Input: dimensioned drawing with shaded views. Units: mm. Origin: part minimum x, y, z. A direction names the side the tool comes from. Give positions to 0.01 mm unless a question says otherwise; leave off trailing zeros. Order: outer loops, then holes, each group sorted by start corner. A loop starts at its lowest first (then second) coordinate and runs counter-clockwise, first axis right, second up. Notation, with made-up numbers: M 7.5,-12 L 13.5,-12 A17 cw 13.5,13 Z; hole C 22,67.5 d4. An arc over 180 degrees is marked long. Answer in a Markdown table with one row per item. Add a question column.
(1) Section query D-D, the plane z = 6. Return loops of the section in (x, y), plus the area to 3 significant figures.
(2) Pin query (flat end, axial travel): P1, Ø15, axis at y = 26, z = 33.5, coming from the +X side; P2, Ø2, axis at y = 29.5, z = 10, coming from the +X side; P3, Ø1, axis at x = 41.5, y = 20.5, coming from the +Z side; P4, Ø6, axis at x = 41, z = 25, coming from the -Y side. Return the tip coordinate at first contact, or that it passes through.
(3) Section query C-C, the plane y = 17.34. Return loops of the section in (x, z), plus the area to 3 significant figures.
(4) Section query A-A, the plane z = 42. Return loops of the section in (x, y).
(5) Section query B-B, the plane x = 30.5. Return loops of the section in (y, z), plus the area to 3 significant figures.
(6) Set-up query: the marked faces 1 and 2. Return all of +Z, -Z, +X, -X, +Y, -Y with unobstructed straight access to the full face (end or side cutting, diameter ignored); none if empty.
(7) Mould query, pull axis Y, two halves, no side actions, for the marked faces 3, 4 and 5. Classes: pulls with the +Y half, pulls with the -Y half, needs draft (parallel to the pull), parting line crosses it, or undercut.
(8) Material intervals for line 1 along Y through (x, z) = (25.5, 5) (3 decimals); line 2 along X through (y, z) = (14, 32.5); line 3 along Z through (x, y) = (41, 16), sorted ascending.
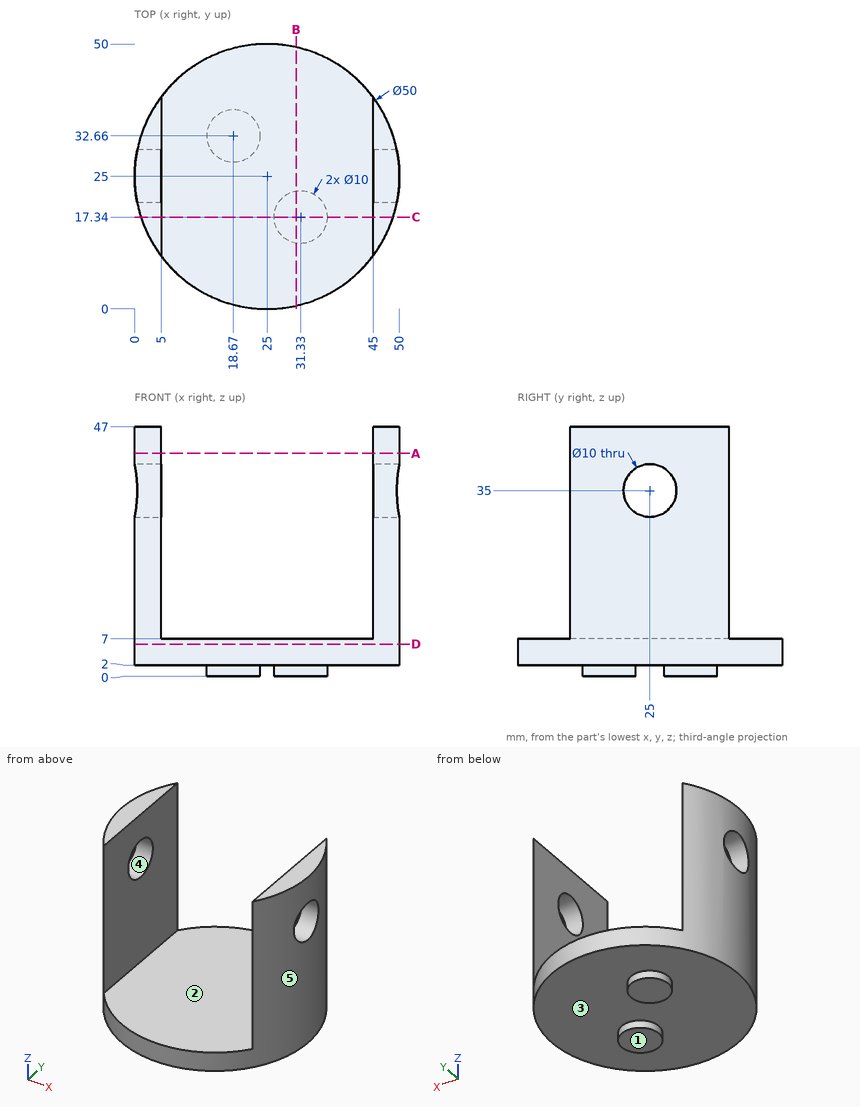
Values follow:
| question | item | result |
|---|---|---|
| 1 | outline | C 25,25 d50 |
| 1 | area | 1,960 mm² |
| 2 | P1 | stops at x = 50 |
| 2 | P2 | stops at x = 49.75 |
| 2 | P3 | stops at z = 7 |
| 2 | P4 | passes through |
| 3 | outline | M 1.2,2 L 26.33,2 L 26.33,0 L 36.33,0 L 36.33,2 L 48.8,2 L 48.8,47 L 45,47 L 45,7 L 5,7 L 5,47 L 1.2,47 Z |
| 3 | area | 562 mm² |
| 4 | outline | M 5,10 L 5,40 A25 ccw Z; M 45,10 A25 ccw 45,40 Z |
| 5 | outline | M 0.61,2 L 12.41,2 L 12.41,0 L 22.27,0 L 22.27,2 L 49.39,2 L 49.39,7 L 0.61,7 Z |
| 5 | area | 264 mm² |
| 6 | face 1 | -Z, +X, -X, +Y, -Y |
| 6 | face 2 | +Z, +Y, -Y |
| 7 | face 3 | needs draft |
| 7 | face 4 | undercut |
| 7 | face 5 | parting line crosses it |
| 8 | line 1 | y = 0.005 to 49.995 |
| 8 | line 2 | x = 2.55 to 5, 45 to 47.45 |
| 8 | line 3 | z = 2 to 7 |
